```python
from build123d import *

# Parameters (mm, degrees)
F0_W     = 762
F0_H     = 812.8
F1_DEPTH = 6.35
F3_DEPTH = 552.45
F4_W     = 647.7000117302
F4_H     = 596.9000117302
F5_DEPTH = 6.35


with BuildPart() as f1:
    # F0 (on Front) → F1 (new body)
    with BuildSketch(Plane.XZ):
        Rectangle(F0_W, F0_H)
    extrude(amount=F1_DEPTH)

    # F2 (on face) → F3 (join)
    with BuildSketch(Plane.XZ.offset(6.35)):
        Polygon((-330.2, -304.8), (330.2, -304.8), (330.2, 298.4500058651), (323.8500058651, 298.4500058651), (323.8500058651, -298.4500058651), (-323.8500058651, -298.4500058651), (-323.8500058651, 298.4500058651), (-330.2, 298.4500058651), align=None)
    extrude(amount=F3_DEPTH)

    # F4 (on face) → F5 (join)
    with BuildSketch(Plane.XZ.offset(558.8)):
        Polygon((-330.2, 298.4500058651), (-330.2, -304.8), (330.2, -304.8), (330.2, 298.4500058651), (323.8500058651, 298.4500058651), (323.8500058651, -298.4500058651), (-323.8500058651, -298.4500058651), (-323.8500058651, 298.4500058651), align=None)
        Rectangle(F4_W, F4_H)
    extrude(amount=F5_DEPTH)


solid = f1.part
```
Verification items for the finished model (mm, model axes). A direction names the side the tool comes from. Round coordinates to 2 decimals unless told otherwise and drop trailing zeros. Order: outer loops, then holes, each group sorted by start corner. A loop starts at its lowest first (then second) coordinate and runs counter-clockwise, first axis right, second up. Notation, with made-up numbers: (-2.75, 27.25) -> (47.25, 27.25) arc R15 cw to (47.25, 35.25) -> close; hole circle Ø10 at (79.5, 18.5). An arc over 180 degrees is marked (long way). Put each result on its own line as item: value. Start each with the question number.
(1) Section check B-B (x = -135). Enter the section's corners in (y, z), then the cut area to 3 significant figures.
(2) Section check C-C (y = -290). Enter the section's corners in (x, z), then the cut area to 3 significant figures.
(3) Depth check by flat-ended pin: pin 1 Ø5 at (x, z) = (100, 230.5) entering from +Y; pin 2 Ø12 at (x, y) = (195, -304.5) entering from +Z; pin 3 Ø6 at (y, z) = (-84.5, -255.5) entering from -X; pin 4 Ø2 at (x, y) = (33, -103.5) entering from -Z. Enter the tip coordinate at first touch or a pass-through.
(4) Section check D-D (z = -318.5). Enter the section's corners in (x, y), then the cut area to 3 significant figures.
(5) Tool access check on faces 1 (the face through (5, -279, -298.45)), 2 (the face through (330.2, -282, -7)), 3 (the face through (-5, -282, -304.8)). Record the directions out of +Z, -Z, +X, -X, +Y, -Y that give a thin tool (end or side, any length) a straight path to the whole face; none if there is none.
(6) Material ranges on line 1 along Y through (x, z) = (-45, 156.5); line 2 along X through (y, z) = (-85, -46.5); line 3 along Z through (x, y) = (-12.5, -493), recorded low to high.
(7) Draft check along Y on faces 4 (the face through (-5, -565.15, 1)), 5 (the face through (-323.85, -279, -4)), 6 (the face through (-5, 0, 6)), 7 (the face through (-330.2, -282, 1)). Enter one of: +Y half, -Y half, draft (parallel to the pull), parting line (faces both ways), or undercut.
(8) Section check A-A (z = 136). Enter the section's corners in (x, y).
Completed:
1. outline: (-565.15, -304.8) -> (-6.35, -304.8) -> (-6.35, -406.4) -> (0, -406.4) -> (0, 406.4) -> (-6.35, 406.4) -> (-6.35, -298.45) -> (-558.8, -298.45) -> (-558.8, 298.45) -> (-565.15, 298.45) -> close
1. area: 12,500 mm2
2. outline: (-330.2, -304.8) -> (330.2, -304.8) -> (330.2, 298.45) -> (323.85, 298.45) -> (323.85, -298.45) -> (-323.85, -298.45) -> (-323.85, 298.45) -> (-330.2, 298.45) -> close
2. area: 11,800 mm2
3. pin 1: stops at y = 0
3. pin 2: stops at z = -298.45
3. pin 3: stops at x = -330.2
3. pin 4: stops at z = -304.8
4. outline: (-381, -6.35) -> (381, -6.35) -> (381, 0) -> (-381, 0) -> close
4. area: 4,840 mm2
5. face 1: +Z
5. face 2: +Z, -Z, +X, -Y
5. face 3: -Z, +X, -X, -Y
6. line 1: y = -565.15 to -558.8, -6.35 to 0
6. line 2: x = -330.2 to -323.85, 323.85 to 330.2
6. line 3: z = -304.8 to -298.45
7. face 4: -Y half
7. face 5: undercut
7. face 6: +Y half
7. face 7: draft
8. outline: (-381, -6.35) -> (-330.2, -6.35) -> (-330.2, -565.15) -> (330.2, -565.15) -> (330.2, -6.35) -> (381, -6.35) -> (381, 0) -> (-381, 0) -> close; hole (-323.85, -558.8) -> (323.85, -558.8) -> (323.85, -6.35) -> (-323.85, -6.35) -> close
